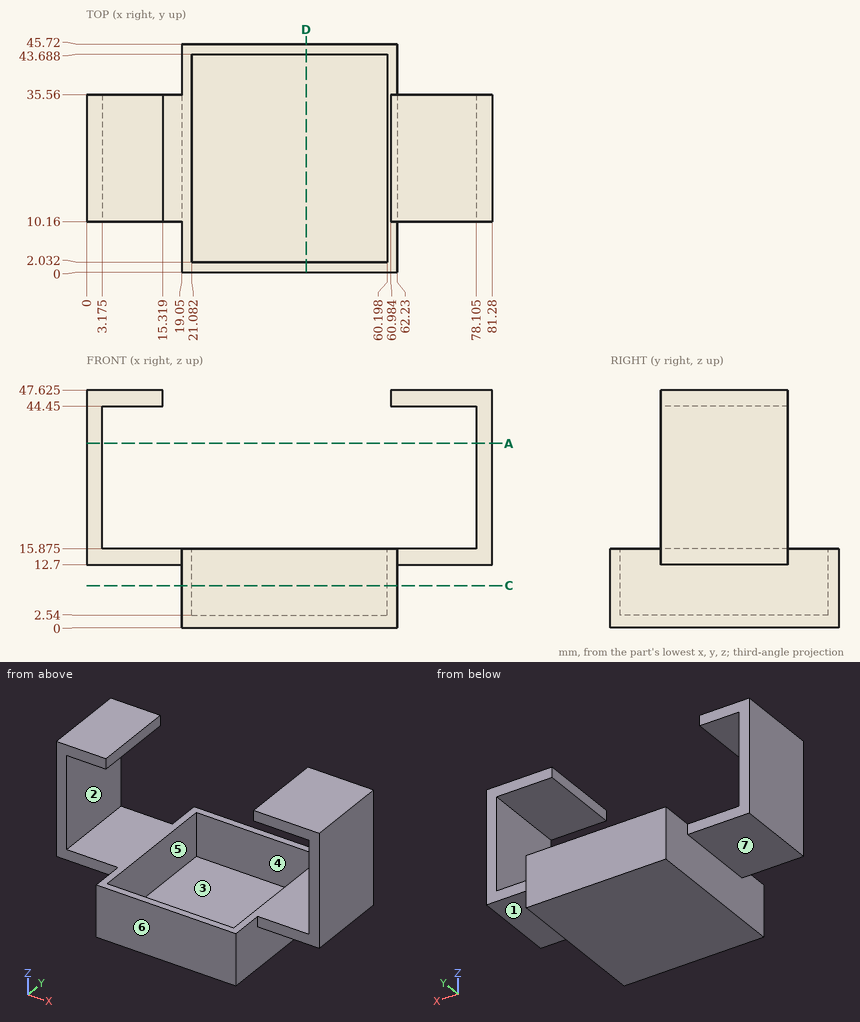
Answer from the drawing. Dimensions are ordinates in mm from the lowest x, y and z of the part. A direction names the side the tool comes from. Coordinates: 2 decimals unless noted, no trailing zeros. Order: outer loops, then holes, each group sorted by start corner. A loop starts at its lowest first (then second) coordinate and runs counter-clockwise, first axis right, second up. Notation, with made-up numbers: (-1, 14) - (27, 14) arc R14 cw to (27, 24) - close; hole circle Ø10 at (53, 49.25). An arc over 180 degrees is marked (long way). Put each result on its own line as item: value. Start each with the question number.
1) Find the intervals of material crossed by line 1 (X direction, y = 22, z = 44) (1 decimal); line 2 (X direction, y = 13.5, z = 10); line 3 (Y direction, x = 53, z = 6), in increasing order. Write a range as from..to.
2) Find section A-A (z = 37). Give the vertices of the cut face in (x, y) (1 decimal).
3) For the marked faces 1, 2 and 3, determine the directions among +Z, -Z, +X, -X, +Y, -Y from which every point of the face is accessible in a straight line to the end or side of a thin tool.
4) For a pull along Y with two mould halves and no side action, classify the marked faces 4, 5, 6 and 7 as released by +Y, released by -Y, zero draft, split by the parting line, or undercut.
5) Find section C-C (z = 8.5). Give the vertices of the cut face in (x, y), plus the area to 3 significant figures.
6) Find section D-D (x = 44). Give the vertices of the cut face in (y, z) (1 decimal), plus the area to 3 significant figures.
7) Flat-ended cylindrical pins translate along their axes: pin 1 (4 mm diameter, centred on y = 13.5, z = 9.5, fed in from +X); pin 2 (4 mm diameter, centred on y = 41, z = 12.5, fed in from -X); pin 3 (5.5 mm diameter, centred on x = 75.5, y = 29, fed in from -Z); pin 4 (1.5 mm diameter, centred on x = 72, z = 10.5, fed in from -Y). Find the tip coordinate at first contact, or state that the pin passes through.
Results list:
1. line 1: x = 0..3.2, 78.1..81.3
1. line 2: x = 19.05..21.08, 60.2..62.23
1. line 3: y = 0..2.03, 43.69..45.72
2. outline: (0, 10.2) - (3.2, 10.2) - (3.2, 35.6) - (0, 35.6) - close; (78.1, 10.2) - (81.3, 10.2) - (81.3, 35.6) - (78.1, 35.6) - close
3. face 1: -Z, +X, +Y, -Y
3. face 2: +Y, -Y
3. face 3: +Z
4. face 4: undercut
4. face 5: undercut
4. face 6: released by -Y
4. face 7: zero draft
5. outline: (19.05, 0) - (62.23, 0) - (62.23, 45.72) - (19.05, 45.72) - close; hole (21.08, 2.03) - (60.2, 2.03) - (60.2, 43.69) - (21.08, 43.69) - close
5. area: 345 mm^2
6. outline: (0, 0) - (45.7, 0) - (45.7, 15.9) - (43.7, 15.9) - (43.7, 2.5) - (2, 2.5) - (2, 15.9) - (0, 15.9) - close
6. area: 170 mm^2
7. pin 1: stops at x = 62.23
7. pin 2: stops at x = 19.05
7. pin 3: stops at z = 12.7
7. pin 4: passes through
